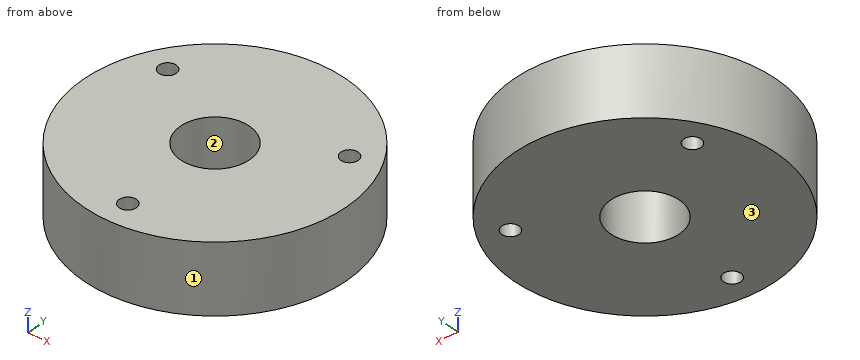
Autodesk Fusion 360 part; units mm, degrees
sketch "Sketch1" plane through (0, 0, 0) normal (0, 0, 1) x (1, 0, 0)
  circle A0 centre (0, 0) radius 10
  circle A1 centre (0, 0) radius 22.5
  circle A2 centre (0, 0) radius 38
  dimension "d1" = 45
  dimension "d2" = 20
  dimension "d3" = 76
extrude "Extrude1" add sketch "Sketch1" along normal blind 20 contours A1
sketch "Sketch2" plane through (0, 0, 0) normal (0, 0, 1) x (1, 0, 0)
  circle A0 centre (0.2654, -30.1553) radius 2.5
  dimension "d8" = 5
extrude "Extrude4" add sketch "Sketch1" along normal blind 2 contours A1 | A2
extrude "Extrude5" cut sketch "Sketch2" along normal blind 6.312
pattern_circular "C-Pattern2" count 3 over 360 about axis through (0, 0, 2) along (0, 0, 1) of "Extrude5"
extrude "돌출6" add 1 faces at (-20.8034, 21.3677, 2) along direction (0, 0, 1) blind 18
The model under review builds one solid part; all positions refer to its coordinate system, in mm. Face numbers are marked on the shaded views. Round coordinates to 2 decimals unless told otherwise and drop trailing zeros. Order: outer loops, then holes, each group sorted by start corner. A loop starts at its lowest first (then second) coordinate and runs counter-clockwise, first axis right, second up. Notation, with made-up numbers: M -21.75,-3.5 L 22.25,-3.5 A17 cw 22.25,5.5 Z; hole C -40,28.25 d6. An arc over 180 degrees is marked long. Use a Markdown table: item, result.
1) Wall thickness on line 1 along X through (y, z) = (-6, 13); line 2 along Y through (x, z) = (-28.5, 16); line 3 along X through (y, z) = (8.5, 12.75): over which ranges is each line inside the solid? List them lowest first. Write a range as [from, to].
Report:
| item | result |
|---|---|
| line 1 | [-37.52, -8], [8, 37.52] |
| line 2 | [-25.13, 13.76], [15.93, 25.13] |
| line 3 | [-37.04, -5.27], [5.27, 37.04] |
2) Consider section A-A (y = 0). Write out the cut boundary in (x, z), then the cut area to 3 significant figures.
Report:
| item | result |
|---|---|
| outline | M -38,0 L -10,0 L -10,20 L -38,20 Z; M 10,0 L 38,0 L 38,20 L 10,20 Z |
| area | 1,120 mm^2 |
3) Insertion check: pin 1 (4 mm diameter, centred on y = -12, z = 14.5, fed in from -X); pin 2 (10 mm diameter, centred on x = 12.5, z = 10.5, fed in from +Y); pin 3 (1 mm diameter, centred on x = -19, z = 6, fed in from +Y); pin 4 (4.5 mm diameter, centred on x = 25.98, y = 15.31, fed in from +Z). Each pin has a flat end and moves straight along its axis. Give the tip position at first contact, or say it passes through.
Report:
| item | result |
|---|---|
| pin 1 | x = -36.66 |
| pin 2 | y = 37.25 |
| pin 3 | y = 33.19 |
| pin 4 | through |
4) Consider section B-B (x = 0). Write out the cut boundary in (y, z), then the cut area to 3 significant figures.
Report:
| item | result |
|---|---|
| outline | M -38,0 L -32.64,0 L -32.64,20 L -38,20 Z; M -27.67,0 L -10,0 L -10,20 L -27.67,20 Z; M 10,0 L 38,0 L 38,20 L 10,20 Z |
| area | 1,020 mm^2 |
5) Consider section C-C (z = 16). Write out the cut boundary in (x, y), then the cut area to 3 significant figures.
Report:
| item | result |
|---|---|
| outline | C 0,0 d76; hole C -26.25,14.85 d5; hole C 0,0 d20; hole C 0.27,-30.16 d5; hole C 25.98,15.31 d5 |
| area | 4,160 mm^2 |
6) Draft analysis for pull direction Y (two halves, no side actions). For the marked faces 1, 2 and 3, state which applies: released by +Y, released by -Y, zero draft, split by the parting line, or undercut.
Report:
| item | result |
|---|---|
| face 1 | split by the parting line |
| face 2 | undercut |
| face 3 | zero draft |
7) Consider section D-D (x = -30). Write out the cut boundary in (y, z).
Report:
| item | result |
|---|---|
| outline | M -23.32,0 L 23.32,0 L 23.32,20 L -23.32,20 Z |
